```python
from build123d import *

# Parameters (mm, degrees)
SKETCH3_W          = 1.016
SKETCH3_H          = 1.016
CHAMFER1_SIZE      = 0.5159375
SKETCH2_R          = 0.762
CUT_EXTRUDE1_DEPTH = 2.54
CHAMFER2_SIZE      = 0.254
CHAMFER2_SIZE_2    = 0.209783356
SKETCH4_OUTSIDE_W  = 21.518
SKETCH4_OUTSIDE_H  = 21.518
CUT_EXTRUDE2_DEPTH = 5.655396081


with BuildPart() as part:
    # Sketch1 → Revolve1 (revolve)
    with BuildSketch(Plane(origin=(0, 0, 0), x_dir=(0, 0, -1), z_dir=(1, 0, 0)), mode=Mode.PRIVATE) as revolve1_sk:
        with BuildLine():
            Line((0, 0), (0, 5.159375))
            Line((0, 5.159375), (-9.525, 5.159375))
            Line((-9.525, 5.159375), (-9.525, 7.14375))
            Line((-9.525, 7.14375), (-11.10615, 7.14375))
            Line((-11.10615, 7.14375), (-11.10615, 3.175))
            Line((-11.10615, 3.175), (-13.586546081, 3.175))
            ThreePointArc((-13.586546081, 3.175), (-15.831610111, 2.24506403), (-16.761546081, 0))
            Line((-16.761546081, 0), (0, 0))
        make_face()
    revolve(revolve1_sk.sketch.rotate(Axis((0, 0, 17.33350529), (0, 0, -1)), 90), axis=Axis((0, 0, 17.33350529), (0, 0, -1)))

    # Sketch3 → Cut-Revolve1 (revolve, cut)
    with BuildSketch(Plane(origin=(0, 0, 0), x_dir=(0, 0, -1), z_dir=(1, 0, 0)), mode=Mode.PRIVATE) as cut_revolve1_sk:
        with Locations((-11.36015, 3.429)):
            Rectangle(SKETCH3_W, SKETCH3_H)
        with Locations((-9.271, 5.413375)):
            Rectangle(SKETCH3_W, SKETCH3_H)
    revolve(cut_revolve1_sk.sketch.rotate(Axis((0, 0, 17.33350529), (0, 0, -1)), 90), axis=Axis((0, 0, 17.33350529), (0, 0, -1)), mode=Mode.SUBTRACT)

    # Chamfer1
    chamfer1_edges = [part.edges().sort_by_distance(p)[0] for p in [
        (-5.159375, 0, 0),
    ]]
    chamfer(chamfer1_edges, length=CHAMFER1_SIZE)

    # Sketch2 → Cut-Extrude1 (cut)
    with BuildSketch(Plane(origin=(0, 0, 0), x_dir=(-1, 0, 0), z_dir=(0, 0, -1))):
        Circle(SKETCH2_R)
    cut_extrude1 = extrude(amount=-CUT_EXTRUDE1_DEPTH, mode=Mode.SUBTRACT)

    # Mirror1: Cut-Extrude1 across plane
    add(cut_extrude1.mirror(Plane.XY.offset(8.38077304)), mode=Mode.SUBTRACT)

    # Chamfer2
    # the kernel refuses this chamfer: 0.254, 0.209783356 mm, written as the material it takes off along each edge
    with BuildSketch(Plane(origin=(0, 0, 0), x_dir=(-1, 0, 0), z_dir=(0, -1, 0))) as chamfer2_piece_1:
        Polygon((0.762 + CHAMFER2_SIZE, 0), (0.762, -CHAMFER2_SIZE), (0.762, 0), align=None)
    revolve(axis=Axis((0, 0, 0), (0, 0, -1)), mode=Mode.SUBTRACT)
    with BuildSketch(Plane(origin=(1e-09, -1e-09, 16.66875), x_dir=(1.0, 1.2724919857814273e-09, -4.6623539153921465e-15), z_dir=(-1.2724919857814273e-09, 1.0, 2.691811803016297e-15))) as chamfer2_piece_2:
        with BuildLine():
            Line((0.997154657, 0.067853643), (0.761999999, CHAMFER2_SIZE_2))
            Line((0.761999999, CHAMFER2_SIZE_2), (0.761999999, 0))
            ThreePointArc((0.761999999, 0), (0.883545151, 0.032618216), (0.997154657, 0.067853643))
        make_face()
    revolve(axis=Axis((1e-09, -1e-09, 16.66875), (0, 0, -1)), revolution_arc=180.000000146, mode=Mode.SUBTRACT)
    with BuildSketch(Plane(origin=(1e-09, 1e-09, 16.66875), x_dir=(-1.0, -1.0948837603327353e-09, 4.6623539045804394e-15), z_dir=(1.0948837603327353e-09, -1.0, -8.075425709502658e-15))) as chamfer2_piece_3:
        with BuildLine():
            Line((0.997154658, 0.067853643), (0.761999999, 0.209783357))
            Line((0.761999999, 0.209783357), (0.762000001, 0))
            ThreePointArc((0.762000001, 0), (0.883545153, 0.032618216), (0.997154658, 0.067853643))
        make_face()
    revolve(axis=Axis((1e-09, 1e-09, 16.66875), (0, 0, -1)), revolution_arc=180.000000125, mode=Mode.SUBTRACT)

    # Sketch4 outside → Cut-Extrude2 (cut)
    with BuildSketch(Plane.XY.offset(16.761546081)):
        Rectangle(SKETCH4_OUTSIDE_W, SKETCH4_OUTSIDE_H)
        Polygon((-2.891420438, 0), (-1.058333333, 3.175), (1.058333333, 3.175), (2.891420438, 0), (1.058333333, -3.175), (-1.058333333, -3.175), align=None, mode=Mode.SUBTRACT)
    extrude(amount=-CUT_EXTRUDE2_DEPTH, mode=Mode.SUBTRACT)


solid = part.part
```
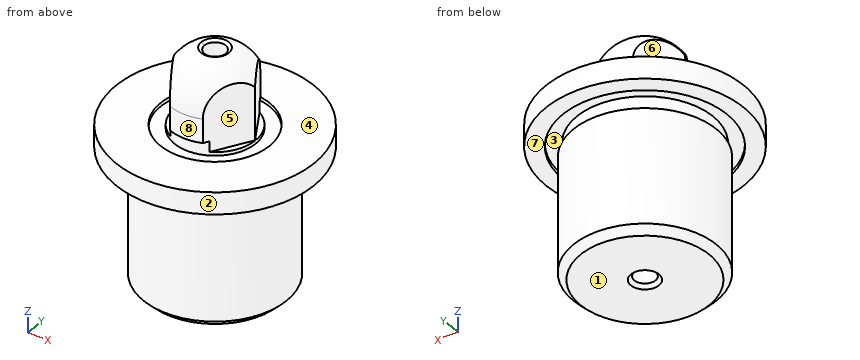
Design review of the part built by this model. Coordinates are the model's own, in mm. Face numbers are marked on the shaded views. A direction names the side the tool comes from. Coordinates: 2 decimals unless noted, no trailing zeros. Order: outer loops, then holes, each group sorted by start corner. A loop starts at its lowest first (then second) coordinate and runs counter-clockwise, first axis right, second up.
1) Take a section at B-B, the plane x = -5.5. Give the boundary of the cut face in (y, z) (3 decimals).
2) Take a section at A-A, the plane z = 14.5. Give the boundary of the cut face in (x, y), and give its area (3 significant figures).
3) Clearance check with flat-ended pins moving along their axes: pin 1 (0.5 mm diameter, centred on x = 0, y = 0, fed in from -Z); pin 2 (6 mm diameter, centred on x = 0.5, z = 4, fed in from -Y); pin 3 (1 mm diameter, centred on x = -2.5, z = 13, fed in from -Y). State where each tip first meets the part, or that it passes through.
4) Wall thickness on line 1 along Y through (x, z) = (0, 10.95); line 2 along Y through (x, z) = (0, 9.7); line 3 along Y through (x, z) = (0, 1.4): over which ranges is each line inside the solid? List them lowest first.
5) For the marked faces 4, 5, 6, 7 and 8, list the 3-axis set-ups (+Z, -Z, +X, -X, +Y, -Y) from which the entire face can be reached by the end or side of a thin tool; tool diameter is ignored.
6) Mouldability with a two-part tool opening along Z and no side actions: class the marked faces 1, 2 and 3 as +Z half, -Z half, draft (parallel to the pull), parting line (faces both ways), or undercut.
7) Take a section at C-C, the plane z = 3. Give the boundary of the cut face in (x, y), and give its area (3 significant figures).
Returned:
1. outline: (-4.559, 9.525) - (-2.194, 9.525) - (-2.194, 9.779) - (2.194, 9.779) - (2.194, 9.525) - (4.559, 9.525) - (4.559, 11.106) - (-4.559, 11.106) - close
2. outline: (-2.89, 0) - (-1.31, -2.75) arc R3.04 ccw to (1.31, -2.75) - (2.89, 0) - (1.31, 2.75) arc R3.04 ccw to (-1.31, 2.75) - close; hole circle Ø1.52 at (0, 0)
2. area: 22.3 mm2
3. pin 1: stops at z = 2.54
3. pin 2: stops at y = -5.16
3. pin 3: stops at y = -1.54
4. line 1: y = -7.14 to -3.94, -2.92 to 2.92, 3.94 to 7.14
4. line 2: y = -7.14 to -5.92, -4.91 to 4.91, 5.92 to 7.14
4. line 3: y = -5.16 to -0.76, 0.76 to 5.16
5. face 4: +Z
5. face 5: +Z, +X, -Y
5. face 6: +Z, -X, +Y
5. face 7: -Z
5. face 8: +Z, -Y
6. face 1: -Z half
6. face 2: draft
6. face 3: undercut
7. outline: circle Ø10.32 at (0, 0)
7. area: 83.6 mm2
